Check sheet for the modelled part. Datum: model origin and axes. Units: mm. A direction names the side the tool comes from. Coordinates: 2 decimals unless noted, no trailing zeros. Write each question's results on one line, items separated by ' | '. Start each with the question number.
from build123d import *

# Parameters (mm, degrees)
SKIZZE1_W                                           = 50
SKIZZE1_H                                           = 50
SKIZZE1_R                                           = 18.55
AUFSATZ_LINEAR_AUSTRAGEN1_DEPTH                     = 21
SKIZZE2_W                                           = 50
SKIZZE2_H                                           = 50
AUFSATZ_LINEAR_AUSTRAGEN2_DEPTH                     = 3
FORMSENKUNG_F_R_M2_5_LINSENSENKSCHRAUBE_D           = 2.7
FORMSENKUNG_F_R_M2_5_LINSENSENKSCHRAUBE_CSINK_D     = 5.5
FORMSENKUNG_F_R_M2_5_LINSENSENKSCHRAUBE_CSINK_ANGLE = 90
SKIZZE5_W                                           = 21
SKIZZE5_H                                           = 46
SCHNITT_LINEAR_AUSTRAGEN1_DEPTH                     = 1
SCHNITT_LINEAR_AUSTRAGEN2_DEPTH                     = 2
SKIZZE7_W                                           = 8
SKIZZE7_H                                           = 12
SCHNITT_LINEAR_AUSTRAGEN3_DEPTH                     = 2.5
KREISMUSTER1_COUNT                                  = 4
SKIZZE8_R                                           = 5
SKIZZE8_R_2                                         = 2.25
AUFSATZ_LINEAR_AUSTRAGEN3_DEPTH                     = 3
FASE1_SIZE                                          = 0.2
FASE1_SIZE2                                         = 0.746410162
SKIZZE10_R                                          = 0.7
SCHNITT_LINEAR_AUSTRAGEN4_DEPTH                     = 5
KREISMUSTER2_COUNT                                  = 4
SCHNITT_LINEAR_START                                = -0.5
SKIZZE12_R                                          = 17.05
SKIZZE12_R_2                                        = 5
SCHNITT_LINEAR_AUSTRAGEN7_DEPTH                     = 0.5
SCHNITT_LINEAR_AUSTRAGEN8_DEPTH                     = 42.12177039
VERRUNDUNG1_R                                       = 1


# Read off the part's stored shape, not the designer's step: Fläche verschieben1
with BuildPart() as part:
    # Skizze1 → Aufsatz-Linear austragen1 (new body)
    with BuildSketch(Plane.XY):
        Rectangle(SKIZZE1_W, SKIZZE1_H)
        with Locations(Location((0, 0, 0), (0, 0, 180))):
            Circle(SKIZZE1_R, mode=Mode.SUBTRACT)
    extrude(amount=AUFSATZ_LINEAR_AUSTRAGEN1_DEPTH)

    # Skizze2 → Aufsatz-Linear austragen2 (add)
    with BuildSketch(Plane.XY.offset(21)):
        Rectangle(SKIZZE2_W, SKIZZE2_H)
    extrude(amount=-AUFSATZ_LINEAR_AUSTRAGEN2_DEPTH)

    # Formsenkung für M2.5 Linsensenkschraube mit Schlitz1 (through all)
    with Locations(Plane.XY.offset(21)):
        with Locations((0, 0)):
            CounterSinkHole(FORMSENKUNG_F_R_M2_5_LINSENSENKSCHRAUBE_D / 2, FORMSENKUNG_F_R_M2_5_LINSENSENKSCHRAUBE_CSINK_D / 2, counter_sink_angle=FORMSENKUNG_F_R_M2_5_LINSENSENKSCHRAUBE_CSINK_ANGLE)

    # Skizze5 → Schnitt-Linear austragen1 (cut)
    with BuildSketch(Plane(origin=(25, 0, 0), x_dir=(0, 0, -1), z_dir=(1, 0, 0))):
        with Locations((-10.5, 0)):
            Rectangle(SKIZZE5_W, SKIZZE5_H)
    schnitt_linear_austragen1 = extrude(amount=-SCHNITT_LINEAR_AUSTRAGEN1_DEPTH, mode=Mode.SUBTRACT)

    # Skizze6 → Schnitt-Linear austragen2 (cut)
    with BuildSketch(Plane(origin=(24, 0, 0), x_dir=(0, 0, -1), z_dir=(1, 0, 0))):
        Polygon((-16, 23), (-21, 18), (-21, -18), (-16, -23), (-5, -23), (0, -18), (0, 18), (-5, 23), align=None)
    schnitt_linear_austragen2 = extrude(amount=-SCHNITT_LINEAR_AUSTRAGEN2_DEPTH, mode=Mode.SUBTRACT)

    # Skizze7 → Schnitt-Linear austragen3 (cut)
    with BuildSketch(Plane(origin=(22, 0, 0), x_dir=(0, 0, -1), z_dir=(1, 0, 0))):
        with Locations((-21, 0)):
            Rectangle(SKIZZE7_W, SKIZZE7_H)
    schnitt_linear_austragen3 = extrude(amount=-SCHNITT_LINEAR_AUSTRAGEN3_DEPTH, mode=Mode.SUBTRACT)

    # Kreismuster1: Schnitt-Linear austragen1, Schnitt-Linear austragen2, Schnitt-Linear austragen3 ×4 about axis
    kreismuster1_axis = Axis((0, 0, 0), (0, 0, 1))
    add([schnitt_linear_austragen1.rotate(kreismuster1_axis, i * 360 / KREISMUSTER1_COUNT) for i in range(1, KREISMUSTER1_COUNT)], mode=Mode.SUBTRACT)
    add([schnitt_linear_austragen2.rotate(kreismuster1_axis, i * 360 / KREISMUSTER1_COUNT) for i in range(1, KREISMUSTER1_COUNT)], mode=Mode.SUBTRACT)
    add([schnitt_linear_austragen3.rotate(kreismuster1_axis, i * 360 / KREISMUSTER1_COUNT) for i in range(1, KREISMUSTER1_COUNT)], mode=Mode.SUBTRACT)

    # Skizze8 → Aufsatz-Linear austragen3 (add)
    with BuildSketch(Plane(origin=(0, 0, 18), x_dir=(-1, 0, 0), z_dir=(0, 0, -1))):
        with Locations(Location((0, 0, 0), (0, 0, 180))):
            Circle(SKIZZE8_R)
        Circle(SKIZZE8_R_2, mode=Mode.SUBTRACT)
    extrude(amount=AUFSATZ_LINEAR_AUSTRAGEN3_DEPTH)

    # Fase1
    fase1_edges = [part.edges().sort_by_distance(p)[0] for p in [
        (2.25, 0, 15),
    ]]
    fase1_side = [part.faces().sort_by_distance(p)[0] for p in [
        (-4.858578644, 0, 15),
    ]]
    chamfer(fase1_edges, length=FASE1_SIZE, length2=FASE1_SIZE2, reference=fase1_side[0])

    # Skizze10 → Schnitt-Linear austragen4 (cut)
    with BuildSketch(Plane(origin=(0, -24, 0), x_dir=(-1, 0, 0), z_dir=(0, -1, 0))):
        with Locations(Location((-21.225, -1.74, 0), (0, 0, 180))):
            Circle(SKIZZE10_R)
        with Locations(Location((21.225, -1.74, 0), (0, 0, 180))):
            Circle(SKIZZE10_R)
        with Locations(Location((21.225, -19.26, 0), (0, 0, 180))):
            Circle(SKIZZE10_R)
        with Locations(Location((-21.225, -19.26, 0), (0, 0, 180))):
            Circle(SKIZZE10_R)
    schnitt_linear_austragen4 = extrude(amount=-SCHNITT_LINEAR_AUSTRAGEN4_DEPTH, mode=Mode.SUBTRACT)

    # Kreismuster2: Schnitt-Linear austragen4 ×4 about axis
    kreismuster2_axis = Axis((0, 0, 0), (0, 0, 1))
    for i in range(1, KREISMUSTER2_COUNT):
        add(schnitt_linear_austragen4.rotate(kreismuster2_axis, i * 360 / KREISMUSTER2_COUNT), mode=Mode.SUBTRACT)

    # Skizze12 → Schnitt-Linear austragen7 (cut)
    with BuildSketch(Plane(origin=(0, 0, 18), x_dir=(-1, 0, 0), z_dir=(0, 0, -1)).offset(SCHNITT_LINEAR_START)):
        Circle(SKIZZE12_R)
        Circle(SKIZZE12_R_2, mode=Mode.SUBTRACT)
    extrude(amount=SCHNITT_LINEAR_AUSTRAGEN7_DEPTH, mode=Mode.SUBTRACT)

    # Fläche verschieben1 outline → Fläche verschieben1 (revolve)
    with BuildSketch(Plane.XZ):
        Polygon((1.35, 18), (1.35, 7), (2.25, 7), (2.25, 4.746410162), (2.45, 4), (5, 4), (5, 7.5), (17.05, 7.5), (17.05, 7), (18.55, 7), (18.55, 18), (17.05, 18), (17.05, 18.5), (5, 18.5), (5, 15), (2.45, 15), (2.25, 15.746410162), (2.25, 18), align=None)
    revolve(axis=Axis((0, 0, 0), (0, 0, 1)))

    # Skizze13 → Schnitt-Linear austragen8 (cut, through all)
    with BuildSketch(Plane.XY.offset(21)):
        with BuildLine():
            ThreePointArc((10.564832878, 4.5425), (0, 11.5), (-10.564832878, 4.5425))
            ThreePointArc((-10.564832878, 4.5425), (-9.779311199, 2.57197832), (-7.808789519, 3.3575))
            ThreePointArc((-7.808789519, 3.3575), (0, 8.5), (7.808789519, 3.3575))
            ThreePointArc((7.808789519, 3.3575), (9.779311199, 2.57197832), (10.564832878, 4.5425))
        make_face()
        with BuildLine():
            ThreePointArc((10.564832878, -4.5425), (0, -11.5), (-10.564832878, -4.5425))
            ThreePointArc((-10.564832878, -4.5425), (-9.779311199, -2.57197832), (-7.808789519, -3.3575))
            ThreePointArc((-7.808789519, -3.3575), (0, -8.5), (7.808789519, -3.3575))
            ThreePointArc((7.808789519, -3.3575), (9.779311199, -2.57197832), (10.564832878, -4.5425))
        make_face()
    extrude(amount=-SCHNITT_LINEAR_AUSTRAGEN8_DEPTH, mode=Mode.SUBTRACT)

    # Verrundung1
    verrundung1_edges = [part.edges().sort_by_distance(p)[0] for p in [
        (9.779311199, 2.57197832, 21),
        (0, 11.5, 21),
        (-9.779311199, 2.57197832, 21),
        (0, 8.5, 21),
        (9.779311199, -2.57197832, 21),
        (0, -8.5, 21),
        (-9.779311199, -2.57197832, 21),
        (0, -11.5, 21),
    ]]
    fillet(verrundung1_edges, radius=VERRUNDUNG1_R)


solid = part.part
Item 1: Section check B-B (z = 9.5). State how many separate pieces and enclosed holes the cut face has, plus the area to 3 significant figures.
Item 2: Release check for a two-part mould opening along Z. For faces 1 (the face through (-21, -23, 3)), 2 (the face through (25, 24, 10)) record: +Z half, -Z half, draft (parallel to the pull), parting line (faces both ways), or undercut.
Item 3: Depth check by flat-ended pin: P1, Ø1.1, axis at y = -21.5, z = 19.5, coming from the +X side; P2, Ø2, axis at x = 21, z = 19, coming from the -Y side; P3, Ø1.3, axis at x = 21.225, z = 1.74, coming from the +Y side. Enter the tip coordinate at first touch or a pass-through.
Item 4: Thickness scan on line 1 (X direction, y = 20.6, z = 19.26); line 2 (Y direction, x = -2, z = 13.5); line 3 (Y direction, x = -4.5, z = 8.5). Record the ranges inside material, lowest first.
Item 5: Tool access check on faces 3 (the face through (0.2, -11.5, 13.8)), 4 (the face through (22.94, -20.557, 19.47)), 5 (the face through (-23, -24, 11)), 6 (the face through (-22.94, 20.557, 19.47)). Record the directions out of +Z, -Z, +X, -X, +Y, -Y that give a thin tool (end or side, any length) a straight path to the whole face; none if there is none.
Computed values:
1) separate pieces: 5 | enclosed holes: 3 | area: 1,790 mm²
2) face 1: undercut | face 2: draft
3) P1: stops at x = 24 | P2: stops at y = -24 | P3: stops at y = 19
4) line 1: x = -19 to -6, 6 to 19 | line 2: y = -22 to -11.32, -8.26 to 8.26, 11.32 to 22 | line 3: y = -22 to -10.58, -7.21 to 7.21, 10.58 to 22
5) face 3: +Z, -Z | face 4: +X | face 5: -Y | face 6: -X
